Autodesk Fusion 360 part; units mm, degrees
sketch "Sketch1" plane through (0, 0, 0) normal (1, 0, 0) x (0, 1, 0)
  circle A0 centre (0, 80) radius 13.595
  dimension "d2" = 27.19
extrude "Extrude1" add sketch "Sketch1" along normal blind 130
sketch "Sketch2" plane through (130, 0, 0) normal (1, 0, 0) x (0, 1, 0)
  circle A0 centre (0, 80) radius 13.595
  line L0 (1.1547, 78) -> (2.3094, 80)
  line L1 (2.3094, 80) -> (1.1547, 82)
  line L2 (1.1547, 82) -> (-1.1547, 82)
  line L3 (-1.1547, 82) -> (-2.3094, 80)
  line L4 (-2.3094, 80) -> (-1.1547, 78)
  line L5 (-1.1547, 78) -> (1.1547, 78)
  point P0 (0, 80)
  dimension "d5" = 2
extrude "Extrude2" add sketch "Sketch2" along normal blind 160 contours L0 L1 L2 L3 L4 L5
chamfer "Chamfer1" distance 1 angle 45 6 edges at (290, -1.7321, 81) (290, 0, 82) (290, -1.7321, 79) (290, 0, 78) (290, 1.7321, 79) (290, 1.7321, 81)
sketch "Sketch3" plane through (130, 0, 0) normal (1, 0, 0) x (0, 1, 0)
  line L0 (-1.1547, 78) -> (-2.3094, 80)
  line L1 (-2.3094, 80) -> (-1.1547, 82)
  line L2 (-1.1547, 82) -> (1.1547, 82)
  line L3 (1.1547, 82) -> (2.3094, 80)
  line L4 (2.3094, 80) -> (1.1547, 78)
  line L5 (1.1547, 78) -> (-1.1547, 78)
  circle A0 centre (0, 80) radius 13.595
sketch "Sketch4" plane through (290, 0, 0) normal (1, 0, 0) x (0, 1, 0)
  line L0 (0.5774, 79) -> (1.1547, 80)
  line L1 (1.1547, 80) -> (0.5774, 81)
  line L2 (0.5774, 81) -> (-0.5774, 81)
  line L3 (-0.5774, 81) -> (-1.1547, 80)
  line L4 (-1.1547, 80) -> (-0.5774, 79)
  line L5 (-0.5774, 79) -> (0.5774, 79)
  line L6 (-0.2, 80.1) -> (-0.2, 82.1)
  line L7 (-0.2, 82.1) -> (-2.8, 82.1)
  line L8 (-2.8, 82.1) -> (-2.8, 80.1)
  line L9 (-2.8, 80.1) -> (-0.2, 80.1)
  line L10 (0.2, 80.1) -> (0.2, 82.1)
  line L11 (0.2, 82.1) -> (2.8, 82.1)
  line L12 (2.8, 82.1) -> (2.8, 80.1)
  line L13 (2.8, 80.1) -> (0.2, 80.1)
  line L14 (0.2, 79.8) -> (2.8, 79.8)
  line L15 (2.8, 79.8) -> (2.8, 77.7841)
  line L16 (2.8, 77.7841) -> (0.2, 77.7841)
  line L17 (0.2, 77.7841) -> (0.2, 79.8)
  line L18 (-0.2, 79.8) -> (-0.2, 77.7841)
  line L19 (-0.2, 77.7841) -> (-2.5, 77.5)
  line L20 (-2.5, 77.5) -> (-2.5, 79.8)
  line L21 (-2.5, 79.8) -> (-0.2, 79.8)
extrude "Extrude3" cut sketch "Sketch4" against normal blind 3 contours L0 L5 L14 L17 | L0 L5 L14 L15 L16 L17 | L4 L5 L18 L19 L20 L21 | L4 L5 L18 L21 | L1 L2 L10 L13 | L1 L2 L10 L11 L12 L13 | L2 L3 L6 L9 | L2 L3 L6 L7 L8 L9
fillet "Fillet1" radius 7.5 1 edges at (130, -12.675, 75.0838)
fillet "Fillet2" radius 10.5 1 edges at (0, -12.675, 75.0838)
equation "diamiter = 27.19 mm"
equation "d2 = diamiter"
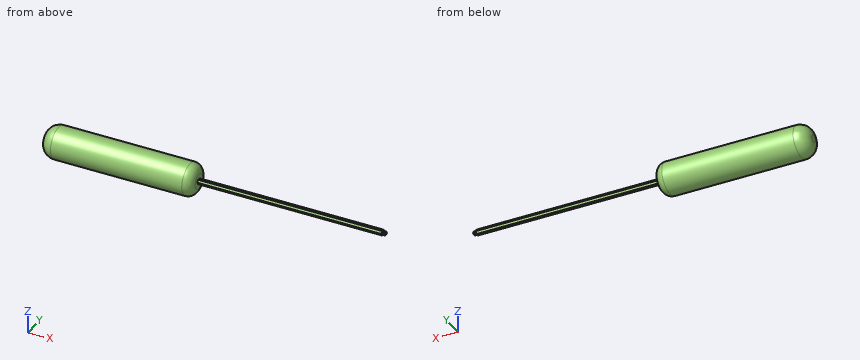
The model under review builds one solid part; all positions refer to its coordinate system, in mm. Round coordinates to 2 decimals unless told otherwise and drop trailing zeros. Loops run counter-clockwise (first coordinate to the right, second up) from the corner with the lowest first, then second, coordinate; pieces in that order, holes last. Notation, with made-up numbers: M 9.5,10 L 14.5,10 A32 ccw 14.5,42 Z; hole C 33.5,10 d7. An arc over 180 degrees is marked long. Answer as CSV lines item,"result". Start each with the question number.
Item 1: Insertion check: P1, Ø8, axis at x = 32.5, z = 86.5, coming from the -Y side; P2, Ø1.8, axis at x = 207.5, y = 0.5, coming from the -Z side; P3, Ø0.5, axis at y = -1.5, z = 78.5, coming from the +X side. Each pin has a flat end and moves straight along its axis. Give the tip position at first contact, or say it passes through.
Item 2: Consider section B-B (x = 107.5). Write out the cut boundary in (y, z) (3 decimals).
Item 3: Consider section A-A (x = 262). Write out the cut boundary in (y, z), then the cut area to 3 significant figures.
Item 4: Wall thickness on line 1 (Y direction, x = 217, z = 80.25); line 2 (Y direction, x = 133.5, z = 80); line 3 (X direction, y = 4.75, z = 86.25): over which ranges is each line inside the solid? List them lowest first. Write a range as [from, to].
Answer:
1,P1,"stops at y = -13.36"
1,P2,"stops at z = 78"
1,P3,"stops at x = 287"
2,outline,"C 0,80 d27.19"
3,outline,"M -2.31,80 L -1.15,78 L 1.15,78 L 2.31,80 L 1.15,82 L -1.15,82 Z"
3,area,"13.9 mm^2"
4,line 1,"y = [-2.17, 2.17]"
4,line 2,"y = [-2.31, 2.31]"
4,line 3,"x = [1.14, 129.79]"
